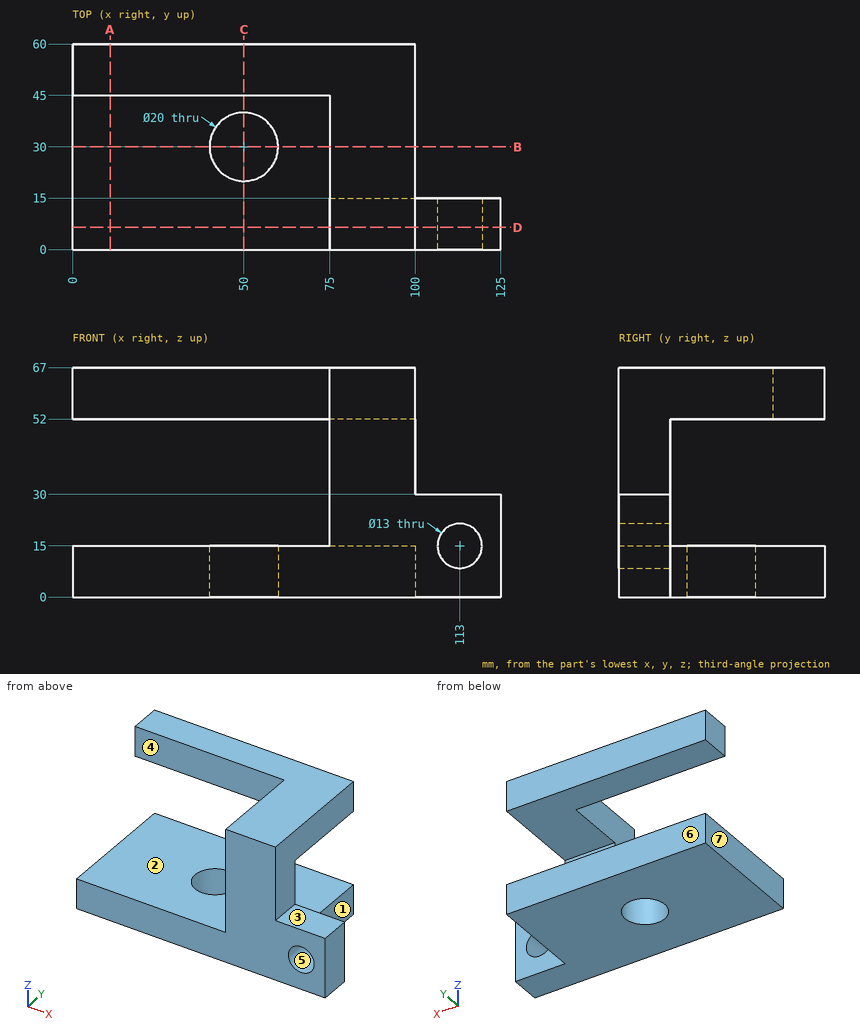
Job drawing, mm, ordinate dimensions from the low corner. One solid piece. A direction names the side the tool comes from. Coordinates: 2 decimals unless noted, no trailing zeros. Write each loop counter-clockwise with the first axis right and the second up, starting at its lowest first coordinate (ties: lowest second). Pieces come first, ordered by that corner, then holes. Notation, with made-up numbers: (72, -20.75) -> (76, -20.75) arc R29 cw to (76, 15.25) -> close; hole circle Ø4 at (29, 51.25). An arc over 180 degrees is marked (long way). Use CSV: the item, a comma, the result in double quotes. Start each with the question number.
Item 1: Band-saw the part on B-B, the plane y = 30. Write the cut outline in (x, z), plus the area to 4 significant figures.
Item 2: Band-saw the part on D-D, the plane y = 6.5. Write the cut outline in (x, z).
Item 3: Drop flat-ended pins along their axis: P1, Ø12, axis at x = 109.5, y = 6.5, coming from the +Z side; P2, Ø1, axis at x = 94.5, y = 15.5, coming from the -Z side; P3, Ø4.5, axis at x = 38, z = 56.5, coming from the -Y side; P4, Ø21, axis at x = 113, z = 15, coming from the +Y side. Give the stop position or say it passes through.
Item 4: Two-plate mould, pull along X, no slides. Class the marked faces 5, 6 and 7: +X half, -X half, draft (parallel to the pull), parting line (faces both ways), or undercut.
Item 5: Wall check: probe 1 along Y at (x, z) = (50, 7); probe 2 along Z at (x, y) = (87.5, 38); probe 3 along Z at (x, y) = (25.5, 27.5). Give the ranges that are in metal, low to high.
Item 6: Band-saw the part on C-C, the plane x = 50. Write the cut outline in (y, z).
Item 7: Band-saw the part on A-A, the plane x = 11. Write the cut outline in (y, z).
Item 8: Tool access for the marked faces 1, 2, 3 and 4: list every direction of +Z, -Z, +X, -X, +Y, -Y with a clear straight run to the whole face (end or side of a thin tool).
Response values:
1,outline,"(0, 0) -> (40, 0) -> (40, 15) -> (0, 15) -> close; (60, 0) -> (100, 0) -> (100, 15) -> (60, 15) -> close; (75, 52) -> (100, 52) -> (100, 67) -> (75, 67) -> close"
1,area,"1,575 mm2"
2,outline,"(0, 0) -> (125, 0) -> (125, 30) -> (100, 30) -> (100, 67) -> (75, 67) -> (75, 15) -> (0, 15) -> close; hole circle Ø13 at (113, 15)"
3,P1,"stops at z = 30"
3,P2,"stops at z = 0"
3,P3,"stops at y = 45"
3,P4,"stops at y = 15"
4,face 5,"undercut"
4,face 6,"draft"
4,face 7,"-X half"
5,probe 1,"y = 0 to 20, 40 to 60"
5,probe 2,"z = 0 to 15, 52 to 67"
5,probe 3,"z = 0 to 15"
6,outline,"(0, 0) -> (20, 0) -> (20, 15) -> (0, 15) -> close; (40, 0) -> (60, 0) -> (60, 15) -> (40, 15) -> close; (45, 52) -> (60, 52) -> (60, 67) -> (45, 67) -> close"
7,outline,"(0, 0) -> (60, 0) -> (60, 15) -> (0, 15) -> close; (45, 52) -> (60, 52) -> (60, 67) -> (45, 67) -> close"
8,face 1,"+Z, -Z, +X, +Y"
8,face 2,"-X, +Y"
8,face 3,"+Z, +X, +Y, -Y"
8,face 4,"+Z, -X, -Y"
